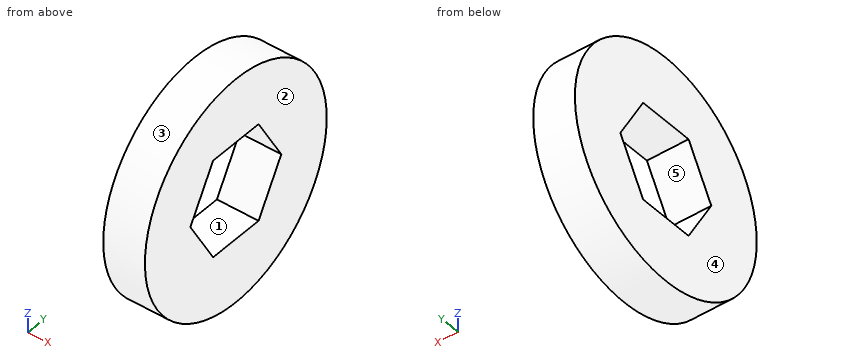
Autodesk Inventor part; units mm, degrees
ref_plane "YZ Plane" through (0, 0, 0) normal (1, 0, 0) x (0, 1, 0)
ref_plane "XZ Plane" through (0, 0, 0) normal (0, 1, 0) x (-1, 0, 0)
ref_plane "XY Plane" through (0, 0, 0) normal (0, 0, 1) x (1, 0, 0)
ref_plane "Work Plane1" through (0, 0, 0) normal (-1, 0, 0) x (0, 0, 1)
sketch "Sketch1" plane through (0, 0, 0) normal (-1, 0, 0) x (0, 0, 1)
  circle A0 centre (0, 0) radius 15
  line L0 (-6.4952, 3.75) -> (-6.4952, -3.75)
  line L1 (0, 7.5) -> (-6.4952, 3.75)
  line L2 (6.4952, 3.75) -> (0, 7.5)
  line L3 (6.4952, -3.75) -> (6.4952, 3.75)
  line L4 (0, -7.5) -> (6.4952, -3.75)
  line L5 (-6.4952, -3.75) -> (0, -7.5)
extrude "Extrusion1" add sketch "Sketch1" along normal blind 5.5
properties part number "wheel_gearing_mount_extension"
Geometry: final body of the model. Coordinates: model frame, mm. Face numbers are marked on the shaded views. A direction names the side the tool comes from. Coordinates: 2 decimals unless noted, no trailing zeros. Write each loop counter-clockwise with the first axis right and the second up, starting at its lowest first coordinate (ties: lowest second). Pieces come first, ordered by that corner, then holes. Notation, with made-up numbers: (82.5, 89) - (130.5, 89) arc R21 cw to (130.5, 126) - close; hole circle Ø6 at (15, 63.25). An arc over 180 degrees is marked (long way). Return JSON: item names as keys, results as strings.
Item 1: Section query B-B (x = -4.3). Output: boundary loops of the cut face in (y, z).
Completed:
{"outline": "circle Ø30 at (0, 0); hole (-7.5, 0) - (-3.75, -6.5) - (3.75, -6.5) - (7.5, 0) - (3.75, 6.5) - (-3.75, 6.5) - close"}
Item 2: Section query A-A (y = 0). Output: boundary loops of the cut face in (x, z), and give its area (3 significant figures).
Completed:
{"outline": "(-5.5, -15) - (0, -15) - (0, -6.5) - (-5.5, -6.5) - close; (-5.5, 6.5) - (0, 6.5) - (0, 15) - (-5.5, 15) - close", "area": "93.6 mm2"}
Item 3: Pull-direction query (Z, two-part tool) for the marked faces 1, 2 and 3; classes: +Z half, -Z half, draft (parallel to the pull), parting line (faces both ways), or undercut.
Completed:
{"face 1": "undercut", "face 2": "draft", "face 3": "parting line"}
Item 4: Pin query (flat end, axial travel): pin 1 Ø1.5 at (x, y) = (-2, 1.5) entering from -Z; pin 2 Ø1.5 at (x, y) = (-3, -10.5) entering from -Z. Return the tip coordinate at first contact, or that it passes through.
Completed:
{"pin 1": "stops at z = -14.98", "pin 2": "stops at z = -11.4"}
Item 5: Section query C-C (z = 5.25). Output: boundary loops of the cut face in (x, y), and give its area (3 significant figures).
Completed:
{"outline": "(-5.5, -14.05) - (0, -14.05) - (0, -4.47) - (-5.5, -4.47) - close; (-5.5, 4.47) - (0, 4.47) - (0, 14.05) - (-5.5, 14.05) - close", "area": "105 mm2"}
Item 6: Line query: L1, parallel to Z at x = -1.55, y = -7.25; L2, parallel to Z at x = -0.75, y = 4.25; L3, parallel to Y at x = -2, z = -1.5. Output: solid intervals per line, ascending.
Completed:
{"L1": "z = -13.13 to -0.43, 0.43 to 13.13", "L2": "z = -14.39 to -5.63, 5.63 to 14.39", "L3": "y = -14.92 to -6.63, 6.63 to 14.92"}
Item 7: Reachability of the marked faces 4 and 5 from +Z, -Z, +X, -X, +Y, -Y: full face, straight path, thin tool, end or side. Return the list, or none.
Completed:
{"face 4": "+Z, -Z, -X, +Y, -Y", "face 5": "+X, -X"}
Item 8: Section query D-D (z = 8.25). Output: boundary loops of the cut face in (x, y).
Completed:
{"outline": "(-5.5, -12.53) - (0, -12.53) - (0, 12.53) - (-5.5, 12.53) - close"}
